Could you check a few things on this model? Use its own coordinates, in mm. A direction names the side the tool comes from. Coordinates: 2 decimals unless noted, no trailing zeros. Loops run counter-clockwise (first coordinate to the right, second up) from the corner with the lowest first, then second, coordinate; pieces in that order, holes last. Notation, with made-up numbers: M 29,70.5 L 67,70.5 A33 ccw 67,107.5 Z; hole C -16,-31 d8. An arc over 180 degrees is marked long. Write each question's results on one line, items separated by ' | '.
```python
from build123d import *

# Parameters (mm, degrees)
ESQUISSE1_W             = 110
ESQUISSE1_H             = 144
BOSS_EXTRU_1_DEPTH      = 6
ESQUISSE2_W             = 10
ESQUISSE2_H             = 6
ENL_V_MAT_EXTRU_1_DEPTH = 182.306370544
ESQUISSE3_R             = 1.5
ENL_V_MAT_EXTRU_2_DEPTH = 182.306370544
ESQUISSE4_R             = 2.995
ESQUISSE4_R_2           = 3
ENL_V_MAT_EXTRU_3_DEPTH = 3


with BuildPart() as part:
    # Esquisse1 → Boss.-Extru.1 (new body)
    with BuildSketch(Plane.XY):
        with Locations((-55, 72)):
            Rectangle(ESQUISSE1_W, ESQUISSE1_H)
    extrude(amount=BOSS_EXTRU_1_DEPTH)

    # Esquisse2 → Enlèv. mat.-Extru.1 (cut, through all)
    with BuildSketch(Plane(origin=(0, 0, 0), x_dir=(-1, 0, 0), z_dir=(0, 0, -1))):
        Polygon((40, 102.5), (40, 72.5), (46, 72.5), (46, 40), (65, 40), (65, 34), (40, 34), (40, 50), (30, 50), (30, 56), (0, 56), (0, 144), (65, 144), (65, 138), (46, 138), (46, 102.5), align=None)
        Polygon((110, 144), (85, 144), (85, 138), (104, 138), (104, 102.5), (110, 102.5), align=None)
        Polygon((110, 72.5), (110, 34), (85, 34), (85, 40), (104, 40), (104, 72.5), align=None)
        with Locations((95, 3)):
            Rectangle(ESQUISSE2_W, ESQUISSE2_H)
        with Locations((35, 3)):
            Rectangle(ESQUISSE2_W, ESQUISSE2_H)
        with Locations((95, 53)):
            Rectangle(ESQUISSE2_W, ESQUISSE2_H)
    extrude(amount=-ENL_V_MAT_EXTRU_1_DEPTH, mode=Mode.SUBTRACT)

    # Esquisse3 → Enlèv. mat.-Extru.2 (cut, through all)
    with BuildSketch(Plane(origin=(0, 0, 0), x_dir=(-1, 0, 0), z_dir=(0, 0, -1))):
        with Locations((43, 87.5)):
            Circle(ESQUISSE3_R)
        with Locations((75, 37)):
            Circle(ESQUISSE3_R)
    extrude(amount=-ENL_V_MAT_EXTRU_2_DEPTH, mode=Mode.SUBTRACT)

    # Esquisse4 → Enlèv. mat.-Extru.3 (cut)
    with BuildSketch(Plane(origin=(0, 0, 0), x_dir=(-1, 0, 0), z_dir=(0, 0, -1))):
        with Locations((43, 87.5)):
            Circle(ESQUISSE4_R)
        with Locations((75, 37)):
            Circle(ESQUISSE4_R_2)
    extrude(amount=-ENL_V_MAT_EXTRU_3_DEPTH, mode=Mode.SUBTRACT)


solid = part.part
```
(1) Imagine slicing it at C-C, the plane x = -75. List the corners of the cut face in (y, z) for me.
Reported:
outline: M 0,0 L 34,0 L 34,3 L 35.5,3 L 35.5,6 L 0,6 Z; M 38.5,3 L 40,3 L 40,0 L 144,0 L 144,6 L 38.5,6 Z
(2) Imagine slicing it at D-D, the plane y = 41.5. List the corners of the cut face in (x, z) for me.
Reported:
outline: M -104,0 L -46,0 L -46,6 L -104,6 Z; M -40,0 L 0,0 L 0,6 L -40,6 Z
(3) Imagine slicing it at B-B, the plane x = -43. List the corners of the cut face in (y, z) for me (3 decimals).
Reported:
outline: M 0,0 L 34,0 L 34,6 L 0,6 Z; M 72.5,0 L 84.505,0 L 84.505,3 L 86,3 L 86,6 L 72.5,6 Z; M 89,3 L 90.495,3 L 90.495,0 L 102.5,0 L 102.5,6 L 89,6 Z
(4) Please list where these lines run through material, in increasing order: probe 1 along Y at (x, z) = (-43, 5.4); probe 2 along Y at (x, z) = (-44, 2.4); probe 3 along X at (y, z) = (87.5, 3.85). Write a range as from..to.
Reported:
probe 1: y = 0..34, 72.5..86, 89..102.5 | probe 2: y = 0..34, 72.5..84.68, 90.32..102.5 | probe 3: x = -110..-44.5, -41.5..-40
(5) Will these pins go through, and if not, where does the flat tip stop? P1, Ø1.5, axis at y = 114, z = 2, coming from the +X side; P2, Ø3, axis at y = 40, z = 3, coming from the -X side; P3, Ø2.5, axis at x = -75, y = 37, coming from the +Z side; P4, Ø3, axis at x = -41.5, z = 4, coming from the -Y side.
Reported:
P1: stops at x = -46 | P2: stops at x = -104 | P3: passes through | P4: stops at y = 0
(6) If we mould it in two halves opening along X, with no side actions, what happens to faces 1 (the flat face through (-104, 56, 3)), 2 (the flat face through (-100, 3, 3)), 3 (the flat face through (-94, 40, 3))? For each: released by +X, released by -X, zero draft, split by the parting line, or undercut.
Reported:
face 1: released by -X | face 2: undercut | face 3: zero draft
(7) Imagine slicing it at A-A, the plane y = 87.5. List the corners of the cut face in (x, z) for me (3 decimals).
Reported:
outline: M -110,0 L -45.995,0 L -45.995,3 L -44.5,3 L -44.5,6 L -110,6 Z; M -41.5,3 L -40.005,3 L -40.005,0 L -40,0 L -40,6 L -41.5,6 Z
(8) Which directions (+Z, -Z, +X, -X, +Y, -Y) give clear straight access to the entire face, cutting with the end or side of a thin tool? Please do faces 4 (the flat face through (-30, 53, 3)), 5 (the flat face through (-85, 37, 3)), 6 (the flat face through (-95, 50, 3)), 7 (the flat face through (-56, 138, 3)).
Reported:
face 4: +Z, -Z, +Y | face 5: +Z, -Z, -X | face 6: +Z, -Z | face 7: +Z, -Z, +X, +Y
